from build123d import *

# Parameters (mm, degrees)
IZIM1_W                     = 42.3
IZIM1_H                     = 42.3
Y_KSEKLIK_EKSTR_ZYON1_DEPTH = 38
PAH1_SIZE                   = 5
IZIM2_R                     = 2
KES_EKSTR_ZYON1_DEPTH       = 5
IZIM3_R                     = 11
Y_KSEKLIK_EKSTR_ZYON2_DEPTH = 2
IZIM4_R                     = 2.5
Y_KSEKLIK_EKSTR_ZYON3_DEPTH = 18


with BuildPart() as part:
    # Çizim1 → Yükseklik-Ekstrüzyon1 (new body)
    with BuildSketch(Plane.XY):
        Rectangle(IZIM1_W, IZIM1_H)
    extrude(amount=Y_KSEKLIK_EKSTR_ZYON1_DEPTH)

    # Pah1
    pah1_edges = [part.edges().sort_by_distance(p)[0] for p in [
        (21.15, -21.15, 19),
        (-21.15, -21.15, 19),
        (-21.15, 21.15, 19),
        (21.15, 21.15, 19),
    ]]
    chamfer(pah1_edges, length=PAH1_SIZE)

    # Çizim2 → Kes-Ekstrüzyon1 (cut)
    with BuildSketch(Plane.XY.offset(38)):
        with Locations((-15.5, 15.5)):
            Circle(IZIM2_R)
        with Locations((15.5, 15.5)):
            Circle(IZIM2_R)
        with Locations((-15.5, -15.5)):
            Circle(IZIM2_R)
        with Locations((15.5, -15.5)):
            Circle(IZIM2_R)
    extrude(amount=-KES_EKSTR_ZYON1_DEPTH, mode=Mode.SUBTRACT)

    # Çizim3 → Yükseklik-Ekstrüzyon2 (add)
    with BuildSketch(Plane.XY.offset(38)):
        Circle(IZIM3_R)
    extrude(amount=Y_KSEKLIK_EKSTR_ZYON2_DEPTH)

    # Çizim4 → Yükseklik-Ekstrüzyon3 (add)
    with BuildSketch(Plane.XY.offset(40)):
        Circle(IZIM4_R)
    extrude(amount=Y_KSEKLIK_EKSTR_ZYON3_DEPTH)


solid = part.part
The model under review builds one solid part; all positions refer to its coordinate system, in mm. A direction names the side the tool comes from. Round coordinates to 2 decimals unless told otherwise and drop trailing zeros. Order: outer loops, then holes, each group sorted by start corner. A loop starts at its lowest first (then second) coordinate and runs counter-clockwise, first axis right, second up. Notation, with made-up numbers: (39.5, 78.5) -> (72.5, 78.5) arc R12 cw to (72.5, 99.5) -> close; hole circle Ø1 at (-30, -0.5). An arc over 180 degrees is marked (long way). Return JSON: item names as keys, results as strings.
1. Take a section at D-D (x = -6.5). Write out the cut boundary in (y, z).
Answer block:
{"outline": "(-21.15, 0) -> (21.15, 0) -> (21.15, 38) -> (8.87, 38) -> (8.87, 40) -> (-8.87, 40) -> (-8.87, 38) -> (-21.15, 38) -> close"}
2. For L1, parallel to Y at x = -15.5, z = 34.15; L2, parallel to Y at x = 15, z = 35, list the stretches that pass through material, from the lowest coordinate up. Write a range as [from, to].
Answer block:
{"L1": "y = [-21.15, -17.5], [-13.5, 13.5], [17.5, 21.15]", "L2": "y = [-21.15, -17.44], [-13.56, 13.56], [17.44, 21.15]"}
3. Take a section at B-B (y = 0). Write out the cut boundary in (x, z), then the cut area to 3 significant figures.
Answer block:
{"outline": "(-21.15, 0) -> (21.15, 0) -> (21.15, 38) -> (11, 38) -> (11, 40) -> (2.5, 40) -> (2.5, 58) -> (-2.5, 58) -> (-2.5, 40) -> (-11, 40) -> (-11, 38) -> (-21.15, 38) -> close", "area": "1,740 mm²"}
4. Insertion check: P1, Ø3.5, axis at x = -15.5, y = 15.5, coming from the +Z side; P2, Ø1.5, axis at x = 14, y = -6, coming from the +Z side. Each pin has a flat end and moves straight along its axis. Give the tip position at first contact, or say it passes through.
Answer block:
{"P1": "stops at z = 33", "P2": "stops at z = 38"}
5. For faces 1 (the face through (-21.15, 0, 19)), 2 (the face through (-15.76, 17.483, 35.535)), list the 3-axis set-ups (+Z, -Z, +X, -X, +Y, -Y) from which the entire face can be reached by the end or side of a thin tool; tool diameter is ignored.
Answer block:
{"face 1": "+Z, -Z, -X, +Y, -Y", "face 2": "+Z"}
6. Take a section at A-A (z = 35.5). Write out the cut boundary in (x, y).
Answer block:
{"outline": "(-21.15, -16.15) -> (-16.15, -21.15) -> (16.15, -21.15) -> (21.15, -16.15) -> (21.15, 16.15) -> (16.15, 21.15) -> (-16.15, 21.15) -> (-21.15, 16.15) -> close; hole circle Ø4 at (-15.5, -15.5); hole circle Ø4 at (-15.5, 15.5); hole circle Ø4 at (15.5, -15.5); hole circle Ø4 at (15.5, 15.5)"}
7. The part is to be moulded in two halves that separate along Y. For faces 3 (the face through (-2.38, -10.74, 38.99)), 4 (the face through (18.7, -18.6, 18.7)), 5 (the face through (-16, -15, 33)), say which applies: +Y half, -Y half, draft (parallel to the pull), parting line (faces both ways), or undercut.
Answer block:
{"face 3": "parting line", "face 4": "-Y half", "face 5": "undercut"}
8. Take a section at C-C (z = 8). Write out the cut boundary in (x, y).
Answer block:
{"outline": "(-21.15, -16.15) -> (-16.15, -21.15) -> (16.15, -21.15) -> (21.15, -16.15) -> (21.15, 16.15) -> (16.15, 21.15) -> (-16.15, 21.15) -> (-21.15, 16.15) -> close"}
